CAD build for the part. Positions are in the model's coordinates, mm. A direction names the side the tool comes from. Round coordinates to 2 decimals unless told otherwise and drop trailing zeros. Write each loop counter-clockwise with the first axis right and the second up, starting at its lowest first coordinate (ties: lowest second). Pieces come first, ordered by that corner, then holes. Notation, with made-up numbers: (68.25, 41.5) - (73.25, 41.5) arc R14 cw to (73.25, 48.5) - close; hole circle Ø6 at (-8.5, 60). An arc over 180 degrees is marked (long way). Answer in a Markdown table with one row per item.
```python
from build123d import *

# Parameters (mm, degrees)
SKETCH1_W                  = 50.0888
SKETCH1_H                  = 39.37
BOSS_EXTRUDE1_DEPTH        = 2.54
SKETCH2_W                  = 44.5008
SKETCH2_H                  = 29.972
BOSS_EXTRUDE2_DEPTH        = 5.842
FILLET1_R                  = 2.54
FILLET2_R                  = 1.27
F_1_6_1_6_DIAMETER_HOLE1_D = 1.6
SKETCH5_W                  = 40.64
SKETCH5_H                  = 25.146
CUT_EXTRUDE1_DEPTH         = 5.842


with BuildPart() as part:
    # Sketch1 → Boss-Extrude1 (new body)
    with BuildSketch(Plane(origin=(0, 0, 0), x_dir=(1, 0, 0), z_dir=(0, 1, 0))):
        with Locations((-39.815086883, 34.57343553)):
            Rectangle(SKETCH1_W, SKETCH1_H)
    extrude(amount=BOSS_EXTRUDE1_DEPTH)

    # Sketch2 → Boss-Extrude2 (add)
    with BuildSketch(Plane(origin=(0, 2.54, 0), x_dir=(1, 0, 0), z_dir=(0, 1, 0))):
        with Locations((-39.815086883, 34.57343553)):
            Rectangle(SKETCH2_W, SKETCH2_H)
    extrude(amount=BOSS_EXTRUDE2_DEPTH)

    # Fillet1
    fillet1_edges = [part.edges().sort_by_distance(p)[0] for p in [
        (-64.859486883, 1.27, -54.25843553),
        (-14.770686883, 1.27, -54.25843553),
        (-14.770686883, 1.27, -14.88843553),
        (-64.859486883, 1.27, -14.88843553),
    ]]
    fillet(fillet1_edges, radius=FILLET1_R)

    # Fillet2
    fillet2_edges = [part.edges().sort_by_distance(p)[0] for p in [
        (-62.065486883, 5.461, -49.55943553),
        (-62.065486883, 5.461, -19.58743553),
        (-17.564686883, 5.461, -19.58743553),
        (-17.564686883, 5.461, -49.55943553),
    ]]
    fillet(fillet2_edges, radius=FILLET2_R)

    # Ø1.6 (1.6) Diameter Hole1 (through all)
    with Locations(Plane(origin=(0, 0, 0), x_dir=(-1, 0, 0), z_dir=(0, -1, 0))):
        with Locations((62.319486883, 17.11093553), (39.815086883, 17.11093553), (17.310686883, 17.11093553), (17.310686883, 52.03593553), (39.815086883, 52.03593553), (62.319486883, 52.03593553)):
            Hole(F_1_6_1_6_DIAMETER_HOLE1_D / 2)

    # Sketch5 → Cut-Extrude1 (cut)
    with BuildSketch(Plane(origin=(0, 8.382, 0), x_dir=(1, 0, 0), z_dir=(0, 1, 0))):
        with Locations((-39.815086883, 34.57343553)):
            Rectangle(SKETCH5_W, SKETCH5_H)
    extrude(amount=-CUT_EXTRUDE1_DEPTH, mode=Mode.SUBTRACT)


solid = part.part
```
Q1. Saw through at C-C on y = 5.75. List the corners of the cut face in (x, z).
Computed:
| item | result |
|---|---|
| outline | (-62.07, -48.29) arc R1.27 ccw to (-60.8, -49.56) - (-18.83, -49.56) arc R1.27 ccw to (-17.56, -48.29) - (-17.56, -20.86) arc R1.27 ccw to (-18.83, -19.59) - (-60.8, -19.59) arc R1.27 ccw to (-62.07, -20.86) - close; hole (-60.14, -47.15) - (-19.5, -47.15) - (-19.5, -22) - (-60.14, -22) - close |
Q2. Saw through at B-B on x = -40. List the corners of the cut face in (y, z), then the cut area to 3 significant figures.
Computed:
| item | result |
|---|---|
| outline | (0, -54.26) - (2.54, -54.26) - (2.54, -52.81) - (0, -52.81) - close; (0, -51.26) - (2.54, -51.26) - (2.54, -49.56) - (8.38, -49.56) - (8.38, -47.15) - (2.54, -47.15) - (2.54, -22) - (8.38, -22) - (8.38, -19.59) - (2.54, -19.59) - (2.54, -17.89) - (0, -17.89) - close; (0, -16.33) - (2.54, -16.33) - (2.54, -14.89) - (0, -14.89) - close |
| area | 120 mm2 |
Q3. Saw through at A-A on z = -45. List the corners of the cut face in (x, y), then the cut area to 3 significant figures.
Computed:
| item | result |
|---|---|
| outline | (-64.86, 0) - (-14.77, 0) - (-14.77, 2.54) - (-17.56, 2.54) - (-17.56, 8.38) - (-19.5, 8.38) - (-19.5, 2.54) - (-60.14, 2.54) - (-60.14, 8.38) - (-62.07, 8.38) - (-62.07, 2.54) - (-64.86, 2.54) - close |
| area | 150 mm2 |
Q4. Flat gauge pins, fed straight in: pin 1 (3 mm diameter, centred on y = 5.5, z = -30.5, fed in from +X); pin 2 (1.8 mm diameter, centred on x = -17.31, z = -52.04, fed in from +Y); pin 3 (1.8 mm diameter, centred on y = 5.5, z = -38, fed in from -X). Where does each tip first touch, or does it go through?
Computed:
| item | result |
|---|---|
| pin 1 | stops at x = -17.56 |
| pin 2 | stops at y = 2.54 |
| pin 3 | stops at x = -62.07 |
Q5. Saw through at D-D on x = -32.5. List the corners of the cut face in (y, z).
Computed:
| item | result |
|---|---|
| outline | (0, -54.26) - (2.54, -54.26) - (2.54, -49.56) - (8.38, -49.56) - (8.38, -47.15) - (2.54, -47.15) - (2.54, -22) - (8.38, -22) - (8.38, -19.59) - (2.54, -19.59) - (2.54, -14.89) - (0, -14.89) - close |
Q6. 3-axis set-ups, long thin cutter, end or side, ignore diameter. For faces 1 (the flat face through (-19.495, 6, -34)), 2 (the flat face through (-40, 5, -19.587)), 3 (the cylindrical face through (-17.947, 5.502, -19.95)): which of +Z, -Z, +X, -X, +Y, -Y reach the whole face in a straight line?
Computed:
| item | result |
|---|---|
| face 1 | +Y |
| face 2 | +Z, +X, -X, +Y |
| face 3 | +Z, +X, +Y |
Q7. Drill centre lines: line 1 (Z direction, x = -27.5, y = 2.75); line 2 (X direction, y = 7.5, z = -28); line 3 (X direction, y = 2.25, z = -52). Where is each one in solid material? Low to high.
Computed:
| item | result |
|---|---|
| line 1 | z = -49.56 to -47.15, -22 to -19.59 |
| line 2 | x = -62.07 to -60.14, -19.5 to -17.56 |
| line 3 | x = -64.84 to -63.12, -61.52 to -40.61, -39.02 to -18.11, -16.51 to -14.79 |
Q8. Pull direction Z, two halves, no side cores. Call faces 4 (the flat face through (-40, 1, -14.888)), 5 (the flat face through (-42, 8.382, -21)), 6 (the flat face through (-40, 6, -22)): released by +Z, released by -Z, zero draft, split by the parting line, or undercut.
Computed:
| item | result |
|---|---|
| face 4 | released by +Z |
| face 5 | zero draft |
| face 6 | undercut |
